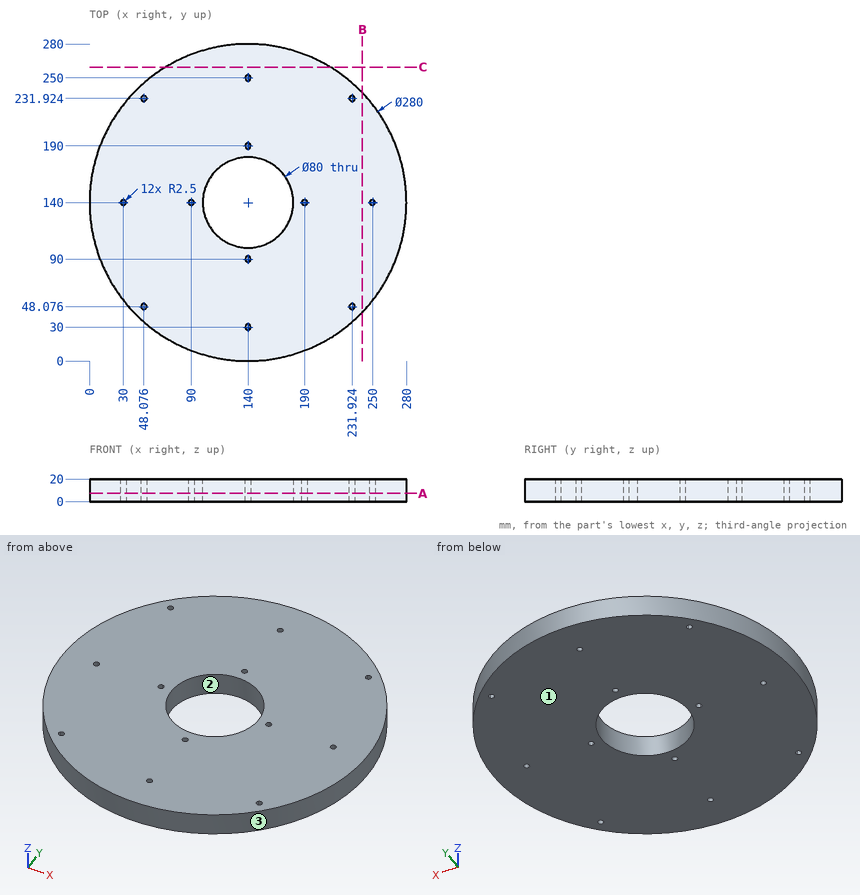
Check sheet for the drawn part. Datum: minimum x, y, z corner. Units: mm. Coordinates: 2 decimals unless noted, no trailing zeros. Order: outer loops, then holes, each group sorted by start corner. A loop starts at its lowest first (then second) coordinate and runs counter-clockwise, first axis right, second up. Notation, with made-up numbers: M 72,89.25 L 96,89.25 A7 cw 96,95.25 Z; hole C -31,-23.75 d6. An arc over 180 degrees is marked long. One line per item, written item: value. Start each with the question number.
Item 1: Gauge pin test, flat ends, axial feed: pin 1 (10 mm diameter, centred on y = 204, z = 15.5, fed in from +X); pin 2 (3 mm diameter, centred on x = 183.5, z = 12, fed in from -Y); pin 3 (1.5 mm diameter, centred on x = 32, z = 9, fed in from -Y). Record the tip position at first contact, or that the pin passes through.
Item 2: Mould release check, pull along Y, two halves, no side actions. Record for the marked faces 1, 2 and 3: released by +Y, released by -Y, zero draft, split by the parting line, or undercut.
Item 3: Scan lines: probe 1 along Y at (x, z) = (140, 8); probe 2 along X at (y, z) = (231, 16); probe 3 along X at (y, z) = (189, 17) (1 decimal). Record each from-to range of solid material in increasing order.
Item 4: Sectioned sample at A-A (z = 7.25). Count the separate pieces of the cut face and the enclosed holes in it, then the cut area to 3 significant figures.
Item 5: Sectioned sample at B-B (x = 241). Enter the section's corners in (y, z), then the cut area to 3 significant figures.
Item 6: Sectioned sample at C-C (y = 259.5). Enter the section's corners in (x, z).
Conclusion:
1. pin 1: stops at x = 266.96
1. pin 2: stops at y = 6.45
1. pin 3: stops at y = 50.01
2. face 1: zero draft
2. face 2: undercut
2. face 3: split by the parting line
3. probe 1: y = 0 to 27.5, 32.5 to 87.5, 92.5 to 100, 180 to 187.5, 192.5 to 247.5, 252.5 to 280
3. probe 2: x = 33.61 to 45.75, 50.4 to 229.6, 234.25 to 246.39
3. probe 3: x = 8.9 to 137.7, 142.3 to 271.1
4. separate pieces: 1
4. enclosed holes: 13
4. area: 56,300 mm^2
5. outline: M 43.05,0 L 236.95,0 L 236.95,20 L 43.05,20 Z
5. area: 3,880 mm^2
6. outline: M 67.06,0 L 212.94,0 L 212.94,20 L 67.06,20 Z
